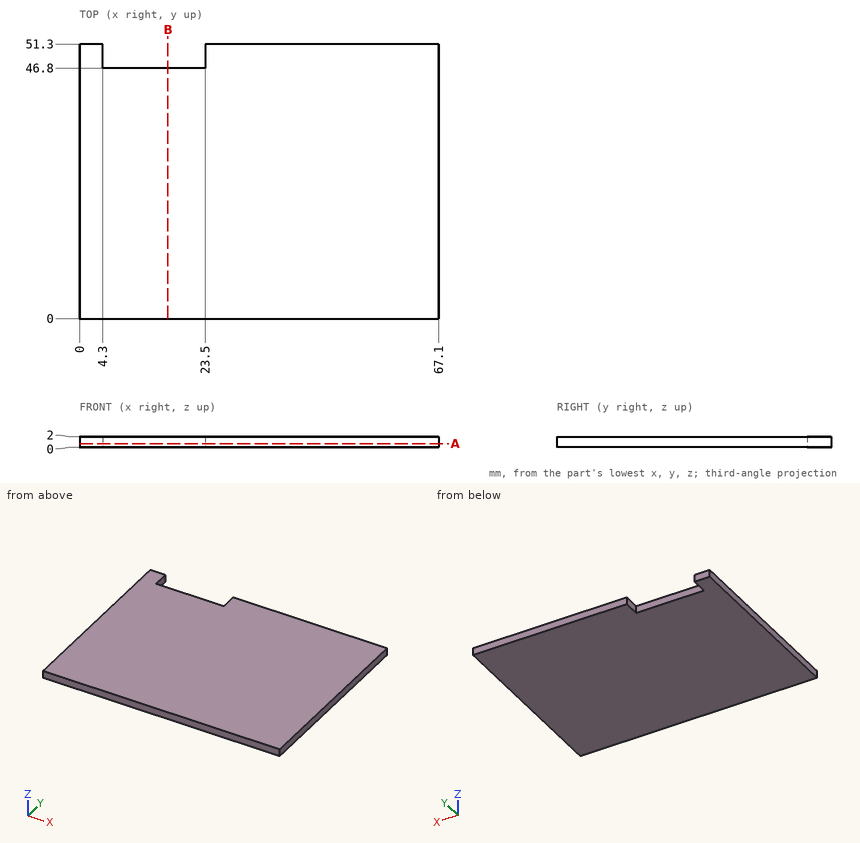
Design review of the part shown in the three views and the two pictorial views. Dimensions are in mm from the part's minimum x, y and z. Coordinates: 2 decimals unless noted, no trailing zeros. Write each loop counter-clockwise with the first axis right and the second up, starting at its lowest first coordinate (ties: lowest second). Pieces come first, ordered by that corner, then holes. Notation, with made-up numbers: (3.25, 11.5) - (35.25, 11.5) arc R26 ccw to (35.25, 46.5) - close; hole circle Ø6 at (47, 88.5). An arc over 180 degrees is marked (long way). Write item = value, one per line.
(1) Consider section B-B, the plane x = 16.5. Give the boundary of the cut face in (y, z), then the cut area to 3 significant figures.
Result sheet:
outline = (0, 0) - (46.8, 0) - (46.8, 2) - (0, 2) - close
area = 93.6 mm^2
(2) For line 1 (X direction, y = 48.5, z = 1.7); line 2 (Y direction, x = 16, z = 0.2), list the stretches that pass through material, from the lowest coordinate up. Write a range as [from, to].
Result sheet:
line_1 = [0, 4.3], [23.5, 67.1]
line_2 = [0, 46.8]
(3) Consider section A-A, the plane z = 0.7. Give the boundary of the cut face in (x, y), then the cut area to 3 significant figures.
Result sheet:
outline = (0, 0) - (67.1, 0) - (67.1, 51.3) - (23.5, 51.3) - (23.5, 46.8) - (4.3, 46.8) - (4.3, 51.3) - (0, 51.3) - close
area = 3,360 mm^2
